Work out the finished part from the listing and answer in its coordinate system (mm). Face numbers are marked on the shaded views. Give positions to 0.01 mm unless a question says otherwise; leave off trailing zeros. Loops run counter-clockwise (first coordinate to the right, second up) from the corner with the lowest first, then second, coordinate; pieces in that order, holes last. Notation, with made-up numbers: (-33.75, -21.5) - (-5.75, -21.5) arc R15 cw to (-5.75, -5.5) - close; hole circle Ø3 at (-9.75, 74). An arc over 180 degrees is marked (long way). Use CSV: the item, a comma, the result in double quotes.
from build123d import *

# Parameters (mm, degrees)
SKETCH1_R           = 0.75
BOSS_EXTRUDE1_DEPTH = 3


with BuildPart() as part:
    # Sketch1 → Boss-Extrude1 (new body)
    with BuildSketch(Plane.XY):
        with BuildLine():
            Line((-0.759056855, 15.743363502), (-10.20503728, 19.025657487))
            ThreePointArc((-10.20503728, 19.025657487), (-11.173300847, 20.75263915), (-9.446319184, 21.720902717))
            Line((-9.446319184, 21.720902717), (0.32477793, 19.593542575))
            Line((0.32477793, 19.593542575), (3.74605929, 18.847766175))
            Line((3.74605929, 18.847766175), (2.548854641, 14.594855726))
            Line((2.548854641, 14.594855726), (-0.759056855, 15.743363502))
        make_face()
        with Locations((-3.96973296, 18.704410315)):
            Circle(SKETCH1_R, mode=Mode.SUBTRACT)
        with Locations((-2.040406529, 18.177438286)):
            Circle(SKETCH1_R, mode=Mode.SUBTRACT)
        with Locations((-0.111080097, 17.650466256)):
            Circle(SKETCH1_R, mode=Mode.SUBTRACT)
        with Locations((1.818246335, 17.123494227)):
            Circle(SKETCH1_R, mode=Mode.SUBTRACT)
    extrude(amount=BOSS_EXTRUDE1_DEPTH)


solid = part.part
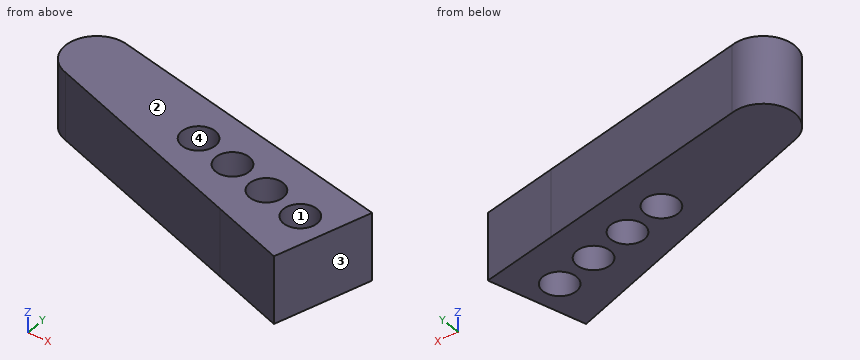
Item 1: A cutting plane is placed at D-D on x = -8.5. Determine the outline of the cut face in (y, z), and give its area (3 significant figures).
Determined:
outline,"(18.43, 0) - (21.51, 0) - (21.51, 3) - (18.43, 3) - close"
area,"9.25 mm²"
Item 2: The mould has two halves that part along X. Classify the marked faces 1, 2, 3 and 4: pulls with the +X half, pulls with the -X half, needs draft (parallel to the pull), parting line crosses it, or undercut.
Determined:
face 1,"undercut"
face 2,"needs draft"
face 3,"pulls with the +X half"
face 4,"undercut"
Item 3: Given P1, Ø1.5, axis at x = -2, z = 2, coming from the +Y side; P2, Ø1.5, axis at x = 1, z = 2, coming from the +Y side, each flat-ended and moving along its own axis, determine where each tip first touches the part or whether it passes through.
Determined:
P1,"stops at y = 20.26"
P2,"stops at y = 19.61"
Item 4: A cutting plane is placed at B-B on y = 19.25. Determine the outline of the cut face in (x, z), and give its area (3 significant figures).
Determined:
outline,"(-10.66, 0) - (-4.48, 0) - (-4.48, 3) - (-10.66, 3) - close; (-3.46, 0) - (1.9, 0) - (1.9, 3) - (-3.46, 3) - close"
area,"34.6 mm²"
Item 5: A cutting plane is placed at C-C on z = 1.05. Determine the outline of the cut face in (x, y).
Determined:
outline,"(-10.21, 19.03) - (-0.76, 15.74) - (2.55, 14.59) - (3.75, 18.85) - (0.32, 19.59) - (-9.45, 21.72) arc R1.4 ccw to start; hole circle Ø1.5 at (-3.97, 18.7); hole circle Ø1.5 at (-2.04, 18.18); hole circle Ø1.5 at (-0.11, 17.65); hole circle Ø1.5 at (1.82, 17.12)"
Item 6: Find the intervals of material crossed by line 1 (Y direction, x = 1.75, z = 2.8); line 2 (Y direction, x = 2, z = 2.7); line 3 (Y direction, x = -7.5, z = 2.85), in increasing order.
Determined:
line 1,"y = 14.87 to 16.38, 17.87 to 19.28"
line 2,"y = 14.79 to 16.4, 17.85 to 19.23"
line 3,"y = 18.09 to 21.3"
Item 7: A cutting plane is placed at A-A on x = -4.25. Determine the outline of the cut face in (y, z).
Determined:
outline,"(16.96, 0) - (18.01, 0) - (18.01, 3) - (16.96, 3) - close; (19.4, 0) - (20.59, 0) - (20.59, 3) - (19.4, 3) - close"
